```python
from build123d import *

# Parameters (mm, degrees)
BOSS_EXTRUDE1_DEPTH = 10
SKETCH1_3_R         = 6
BOSS_EXTRUDE2_DEPTH = 25
SKETCH1_4_R         = 7.5
BOSS_EXTRUDE3_DEPTH = 40
FILLET1_R           = 3
FILLET3_R           = 4
BOSS_EXTRUDE4_START = 105
SKETCH2_R           = 7.5
BOSS_EXTRUDE4_DEPTH = 10
BOSS_EXTRUDE5_START = -115
SKETCH2_2_R         = 7.5
BOSS_EXTRUDE5_DEPTH = 10


with BuildPart() as part:
    # Sketch1 → Boss-Extrude1 (new body)
    with BuildSketch(Plane.XY):
        Polygon((-150, 0), (150, 0), (150, 90), (30, 90), (30, 287.77), (-30, 287.77), (-30, 90), (-150, 90), align=None)
    extrude(amount=BOSS_EXTRUDE1_DEPTH)

    # Sketch1_3 → Boss-Extrude2 (add)
    with BuildSketch(Plane.XY):
        with Locations(Location((0, 195, 0), (0, 0, 180))):
            Circle(SKETCH1_3_R)
    extrude(amount=BOSS_EXTRUDE2_DEPTH)

    # Sketch1_4 → Boss-Extrude3 (add)
    with BuildSketch(Plane.XY):
        with Locations(Location((0, 120, 0), (0, 0, 180))):
            Circle(SKETCH1_4_R)
    extrude(amount=BOSS_EXTRUDE3_DEPTH)

    # Fillet1
    fillet1_edges = [part.edges().sort_by_distance(p)[0] for p in [
        (6, 195, 25),
        (7.5, 120, 40),
    ]]
    fillet(fillet1_edges, radius=FILLET1_R)

    # Fillet3
    fillet3_edges = [part.edges().sort_by_distance(p)[0] for p in [
        (-150, 45, 10),
        (0, 0, 10),
        (150, 45, 10),
        (90, 90, 10),
        (30, 188.885, 10),
        (-30, 188.885, 10),
        (-90, 90, 0),
    ]]
    fillet(fillet3_edges, radius=FILLET3_R)

    # Sketch2 → Boss-Extrude4 (add)
    with BuildSketch(Plane(origin=(0, 0, 0), x_dir=(0, 0, -1), z_dir=(1, 0, 0)).offset(BOSS_EXTRUDE4_START)):
        with BuildLine():
            Line((-10, 67), (-10, 27))
            Line((-10, 27), (-11.76, 27))
            ThreePointArc((-11.76, 27), (-13.004507935, 27.515492065), (-13.52, 28.76))
            Line((-13.52, 28.76), (-13.52, 33.5))
            ThreePointArc((-13.52, 33.5), (-14.984466094, 37.035533906), (-18.52, 38.5))
            Line((-18.52, 38.5), (-30, 38.5))
            ThreePointArc((-30, 38.5), (-38.5, 47), (-30, 55.5))
            Line((-30, 55.5), (-18.52, 55.5))
            ThreePointArc((-18.52, 55.5), (-14.984466094, 56.964466094), (-13.52, 60.5))
            Line((-13.52, 60.5), (-13.52, 65.24))
            ThreePointArc((-13.52, 65.24), (-13.004507935, 66.484507935), (-11.76, 67))
            Line((-11.76, 67), (-10, 67))
        make_face()
        with Locations((-30, 47)):
            Circle(SKETCH2_R, mode=Mode.SUBTRACT)
    extrude(amount=BOSS_EXTRUDE4_DEPTH)

    # Sketch2_2 → Boss-Extrude5 (add)
    with BuildSketch(Plane(origin=(0, 0, 0), x_dir=(0, 0, -1), z_dir=(1, 0, 0)).offset(BOSS_EXTRUDE5_START)):
        with BuildLine():
            Line((-10, 67), (-10, 27))
            Line((-10, 27), (-11.76, 27))
            ThreePointArc((-11.76, 27), (-13.004507935, 27.515492065), (-13.52, 28.76))
            Line((-13.52, 28.76), (-13.52, 33.5))
            ThreePointArc((-13.52, 33.5), (-14.984466094, 37.035533906), (-18.52, 38.5))
            Line((-18.52, 38.5), (-30, 38.5))
            ThreePointArc((-30, 38.5), (-38.5, 47), (-30, 55.5))
            Line((-30, 55.5), (-18.52, 55.5))
            ThreePointArc((-18.52, 55.5), (-14.984466094, 56.964466094), (-13.52, 60.5))
            Line((-13.52, 60.5), (-13.52, 65.24))
            ThreePointArc((-13.52, 65.24), (-13.004507935, 66.484507935), (-11.76, 67))
            Line((-11.76, 67), (-10, 67))
        make_face()
        with Locations((-30, 47)):
            Circle(SKETCH2_2_R, mode=Mode.SUBTRACT)
    extrude(amount=BOSS_EXTRUDE5_DEPTH)


solid = part.part
```
The model under review builds one solid part; all positions refer to its coordinate system, in mm. A direction names the side the tool comes from. Round coordinates to 2 decimals unless told otherwise and drop trailing zeros. Order: outer loops, then holes, each group sorted by start corner. A loop starts at its lowest first (then second) coordinate and runs counter-clockwise, first axis right, second up.
(1) Wall thickness on L1, parallel to X at y = 47, z = 16; L2, parallel to Y at x = -109, z = 30; L3, parallel to X at y = 255, z = 4: over which ranges is each line inside the solid? List them lowest first.
Working result:
L1: x = -115 to -105, 105 to 115
L2: y = 38.5 to 39.5, 54.5 to 55.5
L3: x = -30 to 30
(2) Take a section at D-D, the plane y = 80. State the section outline as (x, z) points, plus the area to 3 significant figures.
Working result:
outline: (-150, 0) - (150, 0) - (150, 6) arc R4 ccw to (146, 10) - (-146, 10) arc R4 ccw to (-150, 6) - close
area: 2,990 mm2
(3) Take a section at B-B, the plane y = 120. State the section outline as (x, z) points, plus the area to 3 significant figures.
Working result:
outline: (-30, 0) - (30, 0) - (30, 6) arc R4 ccw to (26, 10) - (7.5, 10) - (7.5, 37) arc R3 ccw to (4.5, 40) - (-4.5, 40) arc R3 ccw to (-7.5, 37) - (-7.5, 10) - (-26, 10) arc R4 ccw to (-30, 6) - close
area: 1,040 mm2
(4) Tool access review of faces 1 (the face through (-110, 38.5, 24)), 2 (the face through (-115, 47, 18)), 3 (the face through (-110, 55.5, 24)): name each direction out of +Z, -Z, +X, -X, +Y, -Y from which nothing blocks a thin tool from reaching the whole face with its end or side.
Working result:
face 1: +Z, +X, -X, -Y
face 2: +Z, -X, +Y, -Y
face 3: +Z, +X, -X, +Y
(5) Take a section at C-C, the plane x = 68.5. State the section outline as (y, z) points.
Working result:
outline: (0, 0) - (90, 0) - (90, 6) arc R4 ccw to (86, 10) - (4, 10) arc R4 ccw to (0, 6) - close
(6) Take a section at A-A, the plane y = 47. State the section outline as (x, z) points, plus the area to 3 significant figures.
Working result:
outline: (-150, 0) - (150, 0) - (150, 6) arc R4 ccw to (146, 10) - (115, 10) - (115, 22.5) - (105, 22.5) - (105, 10) - (-105, 10) - (-105, 22.5) - (-115, 22.5) - (-115, 10) - (-146, 10) arc R4 ccw to (-150, 6) - close; (-115, 37.5) - (-105, 37.5) - (-105, 38.5) - (-115, 38.5) - close; (105, 37.5) - (115, 37.5) - (115, 38.5) - (105, 38.5) - close
area: 3,260 mm2
(7) Mouldability with a two-part tool opening along X and no side actions: class faces 4 (the face through (105, 47, 18)), 5 (the face through (110, 55.5, 24)), 6 (the face through (-3.461, 126.654, 23.311)) as released by +X, released by -X, zero draft, split by the parting line, or undercut.
Working result:
face 4: undercut
face 5: zero draft
face 6: split by the parting line
(8) For P1, Ø1.4, axis at x = 111, y = 63, coming from the +Z side; P2, Ø5, axis at x = -1, y = 194, coming from the +Z side; P3, Ø5, axis at x = -108, z = 22, coming from the +Y side; P4, Ø2, axis at y = 111, z = 36, coming from the +X side, all flat-tipped, find the tip position at first contact; note any pin that passes through.
Working result:
P1: stops at z = 13.52
P2: stops at z = 25
P3: stops at y = 55.5
P4: passes through
